```python
from build123d import *

# Parameters (mm, degrees)
BOSS_EXTRUDE1_DEPTH = 3
SKETCH2_W           = 3
SKETCH2_H           = 7
CUT_EXTRUDE1_DEPTH  = 10
SKETCH3_R           = 7
SKETCH3_R_2         = 5.302946182
CUT_EXTRUDE2_DEPTH  = 10


with BuildPart() as part:
    # Sketch1 → Boss-Extrude1 (new body)
    with BuildSketch(Plane.XY):
        with BuildLine():
            Line((-20, 52), (20, 52))
            ThreePointArc((20, 52), (44.748737342, 41.748737342), (55, 17))
            Line((55, 17), (55, -28))
            ThreePointArc((55, -28), (43.284271247, -56.284271247), (15, -68))
            Line((15, -68), (0.5, -68))
            Line((0.5, -68), (-0.5, -68))
            Line((-0.5, -68), (-15, -68))
            ThreePointArc((-15, -68), (-43.284271247, -56.284271247), (-55, -28))
            Line((-55, -28), (-55, 17))
            ThreePointArc((-55, 17), (-44.748737342, 41.748737342), (-20, 52))
        make_face()
        with BuildLine():
            Line((-20, 32), (20, 32))
            ThreePointArc((20, 32), (30.606601718, 27.606601718), (35, 17))
            Line((35, 17), (35, -28))
            ThreePointArc((35, -28), (29.142135624, -42.142135624), (15, -48))
            Line((15, -48), (0.5, -48))
            Line((0.5, -48), (-0.5, -48))
            Line((-0.5, -48), (-15, -48))
            ThreePointArc((-15, -48), (-29.142135624, -42.142135624), (-35, -28))
            Line((-35, -28), (-35, 17))
            ThreePointArc((-35, 17), (-30.606601718, 27.606601718), (-20, 32))
        make_face(mode=Mode.SUBTRACT)
    extrude(amount=BOSS_EXTRUDE1_DEPTH)

    # Sketch2 → Cut-Extrude1 (cut)
    with BuildSketch(Plane.XY.offset(3)):
        with Locations((-10.5, 48.5)):
            Rectangle(SKETCH2_W, SKETCH2_H)
        with Locations((-10.5, -64.5)):
            Rectangle(SKETCH2_W, SKETCH2_H)
        with Locations((10.5, -64.5)):
            Rectangle(SKETCH2_W, SKETCH2_H)
        with Locations((10.5, 48.5)):
            Rectangle(SKETCH2_W, SKETCH2_H)
    extrude(amount=-CUT_EXTRUDE1_DEPTH, mode=Mode.SUBTRACT)

    # Sketch3 → Cut-Extrude2 (cut)
    with BuildSketch(Plane.XY.offset(3)):
        with Locations((-45.481132216, 1.090233118)):
            Circle(SKETCH3_R)
        with Locations((-43.578653483, 19.639400767)):
            Circle(SKETCH3_R)
        with Locations((-36.768644381, 35.507802928)):
            Circle(SKETCH3_R)
        with Locations((-21.58124313, 41.57195389)):
            Circle(SKETCH3_R)
        with Locations((-6.718128027, 38.188568416)):
            Circle(SKETCH3_R_2)
        with Locations((-6.718128027, -54.188568416)):
            Circle(SKETCH3_R_2)
        with Locations((-21.58124313, -57.57195389)):
            Circle(SKETCH3_R)
        with Locations((-43.578653483, -35.639400767)):
            Circle(SKETCH3_R)
        with Locations((-45.481132216, -17.090233118)):
            Circle(SKETCH3_R)
        with Locations((45.481132216, -17.090233118)):
            Circle(SKETCH3_R)
        with Locations((43.578653483, -35.639400767)):
            Circle(SKETCH3_R)
        with Locations((21.58124313, -57.57195389)):
            Circle(SKETCH3_R)
        with Locations((6.718128027, -54.188568416)):
            Circle(SKETCH3_R_2)
        with Locations((6.718128027, 38.188568416)):
            Circle(SKETCH3_R_2)
        with Locations((21.58124313, 41.57195389)):
            Circle(SKETCH3_R)
        with Locations((36.768644381, 35.507802928)):
            Circle(SKETCH3_R)
        with Locations((43.578653483, 19.639400767)):
            Circle(SKETCH3_R)
        with Locations((45.481132216, 1.090233118)):
            Circle(SKETCH3_R)
        with Locations((-36.120072086, -49.624208078)):
            Circle(SKETCH3_R)
        with Locations((36.120072086, -49.624208078)):
            Circle(SKETCH3_R)
    extrude(amount=-CUT_EXTRUDE2_DEPTH, mode=Mode.SUBTRACT)


solid = part.part
```
Part model, mm, in its own coordinate system. A direction names the side the tool comes from. Coordinates: 2 decimals unless noted, no trailing zeros. Write each loop counter-clockwise with the first axis right and the second up, starting at its lowest first coordinate (ties: lowest second). Pieces come first, ordered by that corner, then holes.
Item 1: Slice it at B-B (x = 4). Write the cut outline in (y, z).
Item 2: Slice it at D-D (y = -52.5). Write the cut outline in (x, z).
Item 3: Mould opens along Y. For faces 1 (the face through (-36, -7, 0)), 2 (the face through (-28.986, -42.297, 1.479)), 3 (the face through (-42.972, -56.594, 1.479)) say: released by +Y, released by -Y, zero draft, split by the parting line, or undercut.
Item 4: Probe line 1 (Y direction, x = 13.5, z = 1.7); line 2 (X direction, y = 24, z = 2.6); line 3 (Y direction, x = -3, z = 0.85). List the from-to ranges inside material, lowest first.
Item 5: Slice it at C-C (x = 40). Write the cut outline in (y, z), and give its area (3 significant figures).
Item 6: Slice it at A-A (y = -19). Write the cut outline in (x, z), and give its area (3 significant figures).
Item 7: Which spindle directions (+Z, -Z, +X, -X, +Y, -Y) get a long thin tool onto all of the face, cutting with end or side? Do faces 4 (the face through (-16, 52, 1)), 5 (the face through (-35, -6, 1)), 6 (the face through (-9, 48, 2)), 7 (the face through (-12, -65, 2)). Say none if no direction does.
Item 8: Pin check, flat tip, straight feed: pin 1 (0.9 mm diameter, centred on y = 48.5, z = 1, fed in from +X). Stop position of the tip, or through.
Results found:
1. outline: (-68, 0) - (-58.74, 0) - (-58.74, 3) - (-68, 3) - close; (-49.64, 0) - (-48, 0) - (-48, 3) - (-49.64, 3) - close; (32, 0) - (33.64, 0) - (33.64, 3) - (32, 3) - close; (42.74, 0) - (52, 0) - (52, 3) - (42.74, 3) - close
2. outline: (-46.62, 0) - (-42.5, 0) - (-42.5, 3) - (-46.62, 3) - close; (-29.74, 0) - (-26.41, 0) - (-26.41, 3) - (-29.74, 3) - close; (-16.76, 0) - (-11.75, 0) - (-11.75, 3) - (-16.76, 3) - close; (-1.69, 0) - (1.69, 0) - (1.69, 3) - (-1.69, 3) - close; (11.75, 0) - (16.76, 0) - (16.76, 3) - (11.75, 3) - close; (26.41, 0) - (29.74, 0) - (29.74, 3) - (26.41, 3) - close; (42.5, 0) - (46.62, 0) - (46.62, 3) - (42.5, 3) - close
3. face 1: zero draft
3. face 2: undercut
3. face 3: released by -Y
4. line 1: y = -68 to -48, 32 to 52
4. line 2: x = -54.29 to -49.05, -38.1 to -33.27, 33.27 to 38.1, 49.05 to 54.29
4. line 3: y = -68 to -57.97, -50.41 to -48, 32 to 34.41, 41.97 to 52
5. outline: (-59.22, 0) - (-55.45, 0) - (-55.45, 3) - (-59.22, 3) - close; (-43.8, 0) - (-41.66, 0) - (-41.66, 3) - (-43.8, 3) - close; (-29.62, 0) - (-21.44, 0) - (-21.44, 3) - (-29.62, 3) - close; (-12.74, 0) - (-3.26, 0) - (-3.26, 3) - (-12.74, 3) - close; (5.44, 0) - (13.62, 0) - (13.62, 3) - (5.44, 3) - close; (25.66, 0) - (29.3, 0) - (29.3, 3) - (25.66, 3) - close; (41.72, 0) - (45.72, 0) - (45.72, 3) - (41.72, 3) - close
5. area: 118 mm2
6. outline: (-55, 0) - (-52.22, 0) - (-52.22, 3) - (-55, 3) - close; (-38.75, 0) - (-35, 0) - (-35, 3) - (-38.75, 3) - close; (35, 0) - (38.75, 0) - (38.75, 3) - (35, 3) - close; (52.22, 0) - (55, 0) - (55, 3) - (52.22, 3) - close
6. area: 39.2 mm2
7. face 4: +Z, -Z, +X, -X, +Y
7. face 5: +Z, -Z
7. face 6: +Z, -Z, +Y
7. face 7: +Z, -Z, -Y
8. pin 1: stops at x = 36.15
